For this review, take the finished solid that the model builds, in its own axes (mm). A direction names the side the tool comes from. Coordinates: 2 decimals unless noted, no trailing zeros. Write each loop counter-clockwise with the first axis right and the second up, starting at its lowest first coordinate (ties: lowest second). Pieces come first, ordered by that corner, then holes.
1) For faces 1 (the face through (10.3, 21, 3.2)), 2 (the face through (-0.46, 36.05, 19.06)), 3 (the face through (-6.83, 34.32, 12.17)), list the 3-axis set-ups (+Z, -Z, +X, -X, +Y, -Y) from which the entire face can be reached by the end or side of a thin tool; tool diameter is ignored.
2) We need section A-A on z = 3. Write out the cut boundary in (x, y).
3) Insertion check: P1, Ø2, axis at y = 7, z = -9, coming from the +X side; P2, Ø6, axis at y = 23, z = -15, coming from the +X side; P3, Ø2.5, axis at y = 34, z = 0, coming from the -X side; P4, Ø12.5, axis at x = 0, z = 0, coming from the +Y side. Each pin has a flat end and moves straight along its axis. Give the tip position at first contact, or say it passes through.
4) To check wall thickness, follow line 1 along X through (y, z) = (2.5, 9.25); line 2 along Z through (x, y) = (3.5, 34.5); line 3 along Z through (x, y) = (-10, 27). State the ranges of each line that lie inside material, in increasing order.
5) We need section C-C on y = 22. Write out the cut boundary in (x, z), then the cut area to 3 significant figures.
6) We need section B-B on y = 27. Write out the cut boundary in (x, z), then the cut area to 3 significant figures.
7) Mouldability with a two-part tool opening along Y and no side actions: class faces 4 (the face through (19.06, 36.05, 0.46)), 5 (the face through (-5, 0, 15)), 6 (the face through (17.517, 4.979, 10.824)) as pulls with the +Y half, pulls with the -Y half, needs draft (parallel to the pull), parting line crosses it, or undercut.
from build123d import *

# Parameters (mm, degrees)
CIRPATTERN4_COUNT = 6
CIRPATTERN3_COUNT = 12


with BuildPart() as part:
    # Sketch1 → Revolve1 (revolve)
    with BuildSketch(Plane.XY):
        Polygon((12.5, 39), (23, 39), (23, 0), (10.5, 0), (10.5, 24), (12.5, 24), align=None)
    revolve(axis=Axis((0, 64.150553744, 0), (0, 1, 0)))

    # Sketch2 → Cut-Revolve1 (revolve, cut)
    with BuildSketch(Plane.XY):
        Polygon((15, 21), (1, 21), (1, 17), (1, 0), (17, 0), (17, 17), (15, 17), align=None)
    revolve(axis=Axis((1, 17, 0), (0, -1, 0)), mode=Mode.SUBTRACT)

    # Sketch17 → M4x0.7 Tapped Hole1 (revolve, cut)
    with BuildSketch(Plane(origin=(1, 0, 18.5), x_dir=(0, 0, -1), z_dir=(1, 0, 0))):
        Polygon((0, 0), (0, 11.091420021), (1.65, 10.1), (1.65, 0), align=None)
    m4x0_7_tapped_hole1 = revolve(axis=Axis((1, -6.35, 18.5), (0, 1, 0)), mode=Mode.SUBTRACT)

    # CirPattern4: M4x0.7 Tapped Hole1 ×6 about axis
    cirpattern4_axis = Axis((1, 0, 0), (0, 1, 0))
    for i in range(1, CIRPATTERN4_COUNT):
        add(m4x0_7_tapped_hole1.rotate(cirpattern4_axis, i * 360 / CIRPATTERN4_COUNT), mode=Mode.SUBTRACT)

    # Sketch14 → M5x0.8 Tapped Hole1 (revolve, cut)
    with BuildSketch(Plane(origin=(-23, 34, 0), x_dir=(0, 0, 1), z_dir=(0, 1, 0))):
        Polygon((0, 0), (0, 9.2618073), (2.1, 8), (2.1, 0), align=None)
    m5x0_8_tapped_hole1 = revolve(axis=Axis((-29.35, 34, 0), (1, 0, 0)), mode=Mode.SUBTRACT)

    # CirPattern3: M5x0.8 Tapped Hole1 ×12 about axis
    cirpattern3_axis = Axis((0, 64.150553744, 0), (0, -1, 0))
    for i in range(1, CIRPATTERN3_COUNT):
        add(m5x0_8_tapped_hole1.rotate(cirpattern3_axis, i * 360 / CIRPATTERN3_COUNT), mode=Mode.SUBTRACT)


solid = part.part
Result:
1. face 1: -Y
1. face 2: +Z
1. face 3: none
2. outline: (-22.8, 0) - (-14.72, 0) - (-14.72, 17) - (-12.67, 17) - (-12.67, 21) - (-10.06, 21) - (-10.06, 24) - (-12.13, 24) - (-12.13, 39) - (-22.8, 39) - close; (10.06, 21) - (14.67, 21) - (14.67, 17) - (16.72, 17) - (16.72, 0) - (22.8, 0) - (22.8, 39) - (12.13, 39) - (12.13, 24) - (10.06, 24) - close
3. P1: stops at x = 21.56
3. P2: stops at x = 19.62
3. P3: stops at x = -14.49
3. P4: passes through
4. line 1: x = -21.06 to -16.67, -13.37 to -12.06, 14.06 to 15.37, 18.67 to 21.06
4. line 2: z = -22.73 to -12, 12 to 22.73
4. line 3: z = -20.71 to -7.5, 7.5 to 20.71
5. outline: circle Ø46 at (0, 0); hole circle Ø21 at (0, 0)
5. area: 1,320 mm2
6. outline: circle Ø46 at (0, 0); hole circle Ø25 at (0, 0)
6. area: 1,170 mm2
7. face 4: undercut
7. face 5: pulls with the -Y half
7. face 6: needs draft
